Autodesk Inventor part; units mm, degrees
ref_plane "Work Plane6" through (-125, -10, -125) normal (0, 1, 0) x (-1, 0, 0)
ref_plane "YZ Plane" through (0, 0, 0) normal (1, 0, 0) x (0, 1, 0)
ref_plane "XZ Plane" through (0, 0, 0) normal (0, 1, 0) x (-1, 0, 0)
sketch "Sketch1" plane through (0, 0, 0) normal (0, 1, 0) x (-1, 0, 0)
  line L0 (0, 0) -> (250, 0)
  line L1 (250, 0) -> (250, -250)
  line L2 (250, -250) -> (0, -250)
  line L3 (0, -250) -> (0, 0)
  dimension "d0" = 250
  dimension "d1" = 250
extrude "Plate1" add sketch "Sketch1" along normal blind 0.5
sketch "Sketch2" plane through (0, 0.5, 0) normal (0, 1, 0) x (1, 0, 0)
  line L0 (0, 0) -> (-250, 0) construction
  line L1 (0, 250) -> (0, 0) construction
  circle A0 centre (-125, 125) radius 90
  line L2 (-125, 125) -> (-215, 125) construction
  line L3 (-125, 125) -> (-125, 35) construction
  circle A1 centre (-125, 125) radius 87
  dimension "d3" = 125
  dimension "d4" = 125
  dimension "d5" = 180
  dimension "d29" = 3
sketch "Sketch2 outline for Extrusion5" plane through (0, 0.5, 0) normal (0, 1, 0) x (1, 0, 0)
  circle A0 centre (-125, 125) radius 90
extrude "Extrusion5" add sketch "Sketch2 outline for Extrusion5" against normal blind 11 draft -10
extrude "Extrusion6" cut sketch "Sketch2" against normal blind 10.5 draft -10 contours A1
fillet "Fillet1" radius 2.5 4 edges at (-212, 0.5, -125) (-214.9118, 0, -125) (-213.0604, -10.5, -125) (-210.1486, -10, -125)
ref_plane "Work Plane6" through (-125, -10, -125) normal (0, 1, 0) x (-1, 0, 0)
ref_plane "Work Plane5" through (-125, 0.5, -125) normal (0, 1, 0) x (-1, 0, 0)
sketch "Sketch6" plane through (-125, -10, -125) normal (0, 1, 0) x (-1, 0, 0)
  line L0 (0, 0) -> (90, 0) construction
  line L1 (0, 0) -> (0, 90) construction
  arc A0 (60.217391, -8.965909) -> (60.217391, 8.965909) centre (61, 0) ccw
  arc A1 (14.565217, 4.981061) -> (14.565217, -4.981061) centre (15, 0) ccw
  line L2 (14.565217, -4.981061) -> (60.217391, -8.965909)
  line L3 (14.565217, 4.981061) -> (60.217391, 8.965909)
  line L4 (10, 0) -> (70, 0) construction
  arc A2 (2.968884, 15.104379) -> (11.596334, 10.123318) centre (7.5, 12.990381) ccw
  line L5 (2.968884, 15.104379) -> (22.343991, 56.632745)
  line L6 (5, 8.660254) -> (35, 60.621778) construction
  line L7 (11.596334, 10.123318) -> (37.873401, 47.666836)
  arc A3 (37.873401, 47.666836) -> (22.343991, 56.632745) centre (30.5, 52.82755) ccw
  arc A4 (-11.596334, 10.123318) -> (-2.968884, 15.104379) centre (-7.5, 12.990381) ccw
  line L8 (-11.596334, 10.123318) -> (-37.873401, 47.666836)
  line L9 (-5, 8.660254) -> (-35, 60.621778) construction
  line L10 (-2.968884, 15.104379) -> (-22.343991, 56.632745)
  arc A5 (-22.343991, 56.632745) -> (-37.873401, 47.666836) centre (-30.5, 52.82755) ccw
  arc A6 (-14.565217, -4.981061) -> (-14.565217, 4.981061) centre (-15, 0) ccw
  line L11 (-14.565217, -4.981061) -> (-60.217391, -8.965909)
  line L12 (-10, 0) -> (-70, 0) construction
  line L13 (-14.565217, 4.981061) -> (-60.217391, 8.965909)
  arc A7 (-60.217391, 8.965909) -> (-60.217391, -8.965909) centre (-61, 0) ccw
  arc A8 (-2.968884, -15.104379) -> (-11.596334, -10.123318) centre (-7.5, -12.990381) ccw
  line L14 (-2.968884, -15.104379) -> (-22.343991, -56.632745)
  line L15 (-5, -8.660254) -> (-35, -60.621778) construction
  line L16 (-11.596334, -10.123318) -> (-37.873401, -47.666836)
  arc A9 (-37.873401, -47.666836) -> (-22.343991, -56.632745) centre (-30.5, -52.82755) ccw
  arc A10 (11.596334, -10.123318) -> (2.968884, -15.104379) centre (7.5, -12.990381) ccw
  line L17 (11.596334, -10.123318) -> (37.873401, -47.666836)
  line L18 (5, -8.660254) -> (35, -60.621778) construction
  line L19 (2.968884, -15.104379) -> (22.343991, -56.632745)
  arc A11 (22.343991, -56.632745) -> (37.873401, -47.666836) centre (30.5, -52.82755) ccw
  point P0 (-125, 125)
  dimension "d38" = 5
  dimension "d39" = 9
  dimension "d40" = 15
  dimension "d41" = 60
  dimension "d42" = 360
extrude "Extrusion7" cut sketch "Sketch6" against normal blind 0.5
equation "\"d32\" = Profile - Thickness"
equation "\"d34\" = 5 * Thickness"
equation "\"d43\" = Thickness"
equation "\"d2\" = Thickness"
equation "\"BendRadius\" = Thickness"
equation "\"BendReliefWidth\" = Thickness"
equation "\"BendReliefDepth\" = 0.5 * Thickness"
equation "\"CornerReliefSize\" = 4 * Thickness"
equation "\"MinimumRemnant\" = 2 * Thickness"
equation "\"TransitionRadius\" = BendRadius"
equation "\"JacobiRadiusSize\" = BendRadius"
equation "\"GapSize\" = Thickness"
properties part number "A2.2-big-punch-3"
Here's how the part is built. I have some questions about the finished solid (model axes, mm). A direction names the side the tool comes from. Coordinates: 2 decimals unless noted, no trailing zeros. Order: outer loops, then holes, each group sorted by start corner. A loop starts at its lowest first (then second) coordinate and runs counter-clockwise, first axis right, second up.
Item 1: If we mould it in two halves opening along Z, with no side actions, what happens to faces 4 (the face through (-195.227, -8.036, -71.152)), 5 (the face through (-179, 0, -40)), 6 (the face through (-137.52, -10.25, -89.42)), 7 (the face through (-130.09, -10.25, -133.61))? For each: +Z half, -Z half, draft (parallel to the pull), parting line (faces both ways), or undercut.
Result sheet:
face 4: parting line
face 5: draft
face 6: undercut
face 7: undercut
Item 2: For faces 1 (the face through (-126, -10, -126)), 2 (the face through (-137.52, -10.25, -160.58)), 3 (the face through (-126, -10.5, -126)), which set-ups out of +Z, -Z, +X, -X, +Y, -Y let a thin tool reach every point of the face, with its end or its side?
Result sheet:
face 1: +Y
face 2: +Y, -Y
face 3: +Z, -Z, +X, -X, -Y
Item 3: If we section it at D-D on x = -155.5: State how many separate pieces and enclosed holes the cut face has, plus the area to 3 significant figures.
Result sheet:
separate pieces: 4
enclosed holes: 0
area: 159 mm2
Item 4: If we section it at C-C on x = -26: List the corners of the cut face in (y, z) for me, plus the area to 3 significant figures.
Result sheet:
outline: (0, -250) - (0.5, -250) - (0.5, 0) - (0, 0) - close
area: 125 mm2
Item 5: If we section it at B-B on y = -5.25: List the corners of the cut face in (x, z) for me, plus the area to 3 significant figures.
Result sheet:
outline: circle Ø177.97 at (-125, -125); hole circle Ø171.97 at (-125, -125)
area: 1,650 mm2
Item 6: I need wall thicknesses on line 1 (Z direction, x = -94.5, y = -10.25); line 2 (Y direction, x = -179, z = -32); line 3 (Y direction, x = -168, z = -109.5). Which ranges of each line are inside material? Lowest first, please.
Result sheet:
line 1: z = -206.53 to -186.83, -162.13 to -131.37, -118.63 to -87.87, -63.17 to -43.47
line 2: y = 0 to 0.5
line 3: y = -10.5 to -10
Item 7: For P1, Ø11, axis at x = -155.5, z = -177.83, coming from the -Y side; P2, Ø4, axis at x = -42, y = -6.5, coming from the -Z side; P3, Ø4, axis at x = -56, y = -3, coming from the +Z side; P4, Ø23.5, axis at x = -186, z = -125, coming from the +Y side, each with a flat end and sliding along its axis, tell me the tip position at first contact or that it passes through.
Result sheet:
P1: passes through
P2: stops at z = -161.39
P3: stops at z = -65.77
P4: stops at y = -10
Item 8: If we section it at A-A on z = -125: List the corners of the cut face in (x, y) for me, plus the area to 3 significant figures.
Result sheet:
outline: (-250, 0) - (-217.01, 0) arc R2.5 cw to (-214.55, -2.07) - (-213.42, -8.43) arc R2.5 ccw to (-210.96, -10.5) - (-195, -10.5) - (-195, -10) - (-208.05, -10) arc R2.5 cw to (-210.51, -7.93) - (-211.64, -1.57) arc R2.5 ccw to (-214.1, 0.5) - (-250, 0.5) - close; (-135, -10.5) - (-115, -10.5) - (-115, -10) - (-135, -10) - close; (-55, -10.5) - (-39.04, -10.5) arc R2.5 ccw to (-36.58, -8.43) - (-35.45, -2.07) arc R2.5 cw to (-32.99, 0) - (0, 0) - (0, 0.5) - (-35.9, 0.5) arc R2.5 ccw to (-38.36, -1.57) - (-39.49, -7.93) arc R2.5 cw to (-41.95, -10) - (-55, -10) - close
area: 126 mm2
